Autodesk Inventor part; units mm, degrees
ref_plane "YZ Plane" through (0, 0, 0) normal (1, 0, 0) x (0, 1, 0)
ref_plane "XZ Plane" through (0, 0, 0) normal (0, 1, 0) x (-1, 0, 0)
ref_plane "XY Plane" through (0, 0, 0) normal (0, 0, 1) x (1, 0, 0)
sketch "Sketch1" plane through (0, 0, 0) normal (0, 1, 0) x (-1, 0, 0)
  line L0 (18, 9) -> (-18, 9)
  line L1 (-18, 9) -> (-18, -9)
  line L2 (-18, -9) -> (18, -9)
  line L3 (18, -9) -> (18, 9)
  line L4 (18, 9) -> (-18, -9) construction
  line L5 (-18, 9) -> (18, -9) construction
  point P0 (0, 0)
  dimension "d0" = 18
  dimension "d1" = 36
extrude "Extrusion1" add sketch "Sketch1" along normal blind 4
sketch "Sketch2" plane through (18, 0, 9) normal (1, 0, 0) x (0, 0, -1)
  line L0 (3, 9.8571) -> (15, 9.8571)
  line L1 (15, 9.8571) -> (15, 0)
  line L2 (15, 0) -> (3, 0)
  line L3 (3, 0) -> (3, 9.8571)
  line L4 (0.7991, 7.2165) -> (12.7991, -2.6406) construction
  line L5 (12.7991, 7.2165) -> (0.7991, -2.6406) construction
  line L6 (9, 0) -> (9, 4.0958)
  line L7 (9, 0) -> (15, 0)
  line L8 (0, 0) -> (18, 0)
  point P0 (6.7991, 2.2879)
  dimension "d4" = 12
  dimension "d22" = 6
extrude "Extrusion2" cut sketch "Sketch2" against normal blind 34
sketch "Sketch3" plane through (-16, 0, 9) normal (1, 0, 0) x (0, 0, -1)
  line L0 (3, 4) -> (15, 4)
  line L1 (15, 4) -> (15, 0)
  line L2 (3, 4) -> (15, 4)
  line L3 (15, 4) -> (15, 3)
  line L4 (15, 3) -> (3, 3)
  line L5 (3, 3) -> (3, 4)
  point P0 (9, 0)
  dimension "d7" = 1
extrude "Extrusion3" add sketch "Sketch3" along normal blind 3
sketch "Sketch4" plane through (-16, 3, -6) normal (0, -1, 0) x (1, 0, 0)
  line L0 (0, 12) -> (3, 12)
  line L1 (1.5, 12) -> (1.5, 0)
  line L2 (3, 0) -> (0, 0)
  line L3 (3, 0) -> (3, 12)
  line L4 (3, 6) -> (0, 6)
  line L5 (0, 0) -> (0, 12)
  circle A0 centre (1.5, 6) radius 0.95
  point P0 (16, 6)
  dimension "d10" = 1.9
extrude "Extrusion4" add sketch "Sketch4" along normal blind 2.5 contours A0 L4 L1 | L1 L4 A0 | L4 L1 A0 | L4 A0 L1
sketch "Sketch5" plane through (-18, 0, -9) normal (-1, 0, 0) x (0, 0, 1)
  line L0 (18, 0) -> (15, 0)
  line L1 (0, 0) -> (0, 4)
  line L2 (18, 0) -> (0, 0)
  line L3 (0, 0) -> (0, 1)
  line L4 (0, 1) -> (18, 1)
  line L5 (18, 1) -> (18, 0)
  point P0 (9, 0)
  dimension "d13" = 1
extrude "Extrusion5" add sketch "Sketch5" along normal blind 5
sketch "Sketch6" plane through (-18, 1, 9) normal (0, 1, 0) x (1, 0, 0)
  line L0 (0, 18) -> (0, 0)
  circle A0 centre (-2.4881, 9) radius 2.35
  line L1 (36, 18) -> (-5, 18)
  line L2 (-5, 18) -> (0, 18)
  line L3 (-2.5, 18) -> (-2.5, 0)
  line L4 (-5, 0) -> (-5, 18)
  line L5 (-5, 9) -> (0, 9)
  point P0 (18, 9)
  dimension "d17" = 4.7
extrude "Extrusion6" add sketch "Sketch6" against normal blind 40 contours L5 L3 A0 | A0 L3 L5 | L3 L5 A0 | A0 L5 L3
sketch "Sketch7" plane through (-18, 1, 9) normal (0, 1, 0) x (1, 0, 0)
  line L0 (0, 0) -> (-5, 0)
  line L1 (-5, 18) -> (-5, 0)
  line L2 (0, 0) -> (-5, 0)
  line L3 (-5, 0) -> (-5, 18)
  line L4 (-5, 18) -> (0, 18)
  line L5 (0, 18) -> (0, 0)
  point P0 (18, 9)
extrude "Extrusion7" add sketch "Sketch7" along normal blind 3
properties part number "ServoHållare"
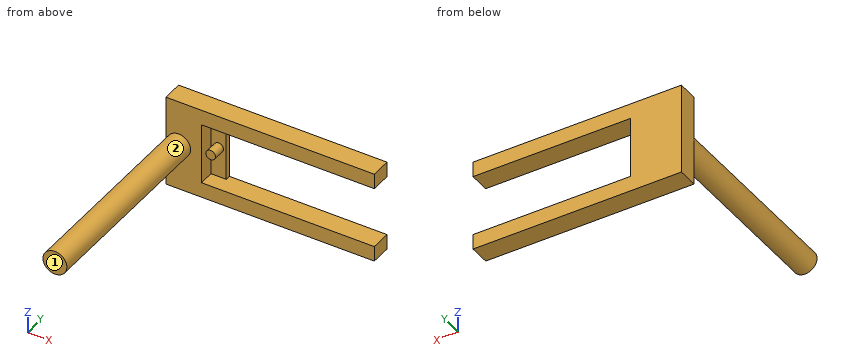
Could you check a few things on this model? Use its own coordinates, in mm. Face numbers are marked on the shaded views. A direction names the side the tool comes from. Coordinates: 2 decimals unless noted, no trailing zeros. Write each loop counter-clockwise with the first axis right and the second up, starting at its lowest first coordinate (ties: lowest second). Pieces come first, ordered by that corner, then holes. Notation, with made-up numbers: (33, 71) - (58, 71) arc R18 ccw to (58, 77) - close; hole circle Ø6 at (53.5, -38.5). An arc over 180 degrees is marked (long way). Write item = value, one per line.
1) Suppose I cut it at D-D on y = -33.5. Please give me the cut outline in (x, z), plus the area to 3 significant figures.
Result set:
outline = circle Ø4.7 at (-20.49, 0)
area = 17.3 mm2
2) For the marked faces 1 and 2, which set-ups out of +Z, -Z, +X, -X, +Y, -Y let a thin tool reach every point of the face, with its end or its side?
Result set:
face_1 = +Z, -Z, +X, -X, -Y
face_2 = -Y
3) Suppose I cut it at B-B on z = 0. Please give me the cut outline in (x, y).
Result set:
outline = (-23, 0) - (-22.84, 0) - (-22.84, -39) - (-18.14, -39) - (-18.14, 0) - (-16, 0) - (-16, 3) - (-15.45, 3) - (-15.45, 0.5) - (-13.55, 0.5) - (-13.55, 3) - (-13, 3) - (-13, 4) - (-23, 4) - close
4) Please list where these lines run through material, in increasing order: line 1 (Z direction, x = 0.5, y = 1.5); line 2 (Z direction, x = -20.5, y = -22); line 3 (Y direction, x = 8, z = 8). Write a range as [from, to].
Result set:
line_1 = [-9, -6], [6, 9]
line_2 = [-2.35, 2.35]
line_3 = [0, 4]
5) Will these pins go through, and if not, where does the flat tip stop? pin 1 Ø2.5 at (y, z) = (1, 1.5) entering from +X; pin 2 Ø1.5 at (x, z) = (-14, 0) entering from -Y; pin 3 Ø6 at (y, z) = (-12, 0.5) entering from +X.
Result set:
pin_1 = -13.58
pin_2 = 0.5
pin_3 = -18.14
6) Suppose I cut it at C-C on x = -14.5. Please give me the cut outline in (y, z), plus the area to 4 significant figures.
Result set:
outline = (0, -9) - (4, -9) - (4, 9) - (0, 9) - (0, 6) - (3, 6) - (3, 0.95) - (0.5, 0.95) - (0.5, -0.95) - (3, -0.95) - (3, -6) - (0, -6) - close
area = 40.75 mm2
7) Suppose I cut it at A-A on x = -8.5. Please give me the cut outline in (y, z).
Result set:
outline = (0, -9) - (4, -9) - (4, -6) - (0, -6) - close; (0, 6) - (4, 6) - (4, 9) - (0, 9) - close
